Read the model definition and answer for the solid it produces. Units are mm, in the model's axes. Face numbers are marked on the shaded views. A direction names the side the tool comes from. Give positions to 0.01 mm unless a question says otherwise; leave off trailing zeros. Order: outer loops, then holes, each group sorted by start corner. A loop starts at its lowest first (then second) coordinate and runs counter-clockwise, first axis right, second up. Notation, with made-up numbers: M -5,0.5 L 48,0.5 A12 ccw 48,22.5 Z; hole C 18.5,10 d6. An arc over 180 degrees is marked long. One line per item, written item: value. Start each with the question number.
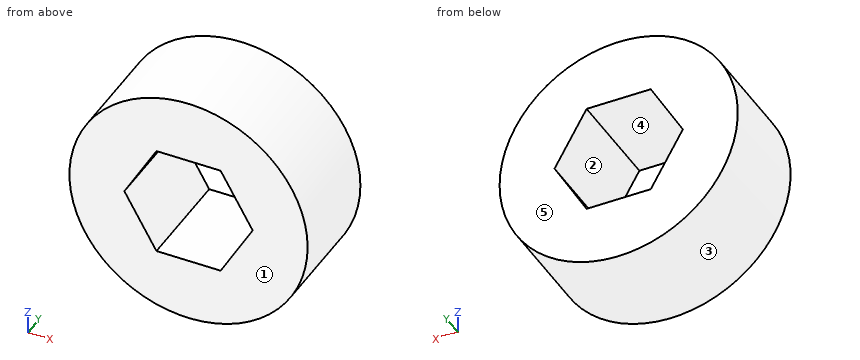
from build123d import *

# Parameters (mm, degrees)
SKETCH1_R               = 15
BOSS_EXTRUDE1_DEPTH     = 13
CUT_EXTRUDE1_DEPTH      = 26
CUT_EXTRUDE1_DEPTH_BACK = 32


with BuildPart() as part:
    # Sketch1 → Boss-Extrude1 (new body)
    with BuildSketch(Plane(origin=(0, 0, 0), x_dir=(1, 0, 0), z_dir=(0, 1, 0))):
        Circle(SKETCH1_R)
    extrude(amount=BOSS_EXTRUDE1_DEPTH)

    # Sketch3 → Cut-Extrude1 (cut, two sides)
    with BuildSketch(Plane(origin=(0, 13, 0), x_dir=(1, 0, 0), z_dir=(0, 1, 0))) as cut_extrude1_sk:
        Polygon((8.082903769, 0), (4.041451884, 7), (-4.041451884, 7), (-8.082903769, 0), (-4.041451884, -7), (4.041451884, -7), align=None)
    extrude(amount=CUT_EXTRUDE1_DEPTH, mode=Mode.SUBTRACT)
    extrude(cut_extrude1_sk.sketch, amount=-CUT_EXTRUDE1_DEPTH_BACK, mode=Mode.SUBTRACT)


solid = part.part
Q1. Consider probe 1 along Z at (x, y) = (1, 8.25); probe 2 along X at (y, z) = (7, 1); probe 3 along X at (y, z) = (7, -3). Determine where each line is inside the solid, lowest interval first.
Q2. A tool of negligible diameter and unlimited length cuts with its end or side. For the marked faces 1 and 2, from which of +Z, -Z, +X, -X, +Y, -Y can it reach the whole face along a straight path? Write none if from no direction.
Q3. This flat-tipped pin is pushed along its axis until it touches: pin 1 (1.5 mm diameter, centred on x = 2, y = 11.5, fed in from -Z). Where does it stop, or does it pass through?
Q4. Find section C-C, the plane y = 6. Give the vertices of the cut face in (x, z), then the cut area to 3 significant figures.
Q5. Find section D-D, the plane x = 12. Give the vertices of the cut face in (y, z).
Q6. Find section B-B, the plane z = 6.25. Give the vertices of the cut face in (x, y).
Q7. Determine the mould class of the marked faces 3, 4 and 5 for opening direction Z: released by +Z, released by -Z, zero draft, split by the parting line, or undercut.
Q8. Find section A-A, the plane x = 0. Give the vertices of the cut face in (y, z), then the cut area to 3 significant figures.
Evaluation:
1. probe 1: -14.97 to -7, 7 to 14.97
1. probe 2: -14.97 to -7.51, 7.51 to 14.97
1. probe 3: -14.7 to -6.35, 6.35 to 14.7
2. face 1: +Z, -Z, +X, -X, -Y
2. face 2: +Y, -Y
3. pin 1: z = -14.95
4. outline: C 0,0 d30; hole M -8.08,0 L -4.04,-7 L 4.04,-7 L 8.08,0 L 4.04,7 L -4.04,7 Z
4. area: 537 mm2
5. outline: M 0,-9 L 13,-9 L 13,9 L 0,9 Z
6. outline: M -13.64,0 L -4.47,0 L -4.47,13 L -13.64,13 Z; M 4.47,0 L 13.64,0 L 13.64,13 L 4.47,13 Z
7. face 3: split by the parting line
7. face 4: undercut
7. face 5: zero draft
8. outline: M 0,-15 L 13,-15 L 13,-7 L 0,-7 Z; M 0,7 L 13,7 L 13,15 L 0,15 Z
8. area: 208 mm2
